Here's how the part is built. I have some questions about the finished solid (model axes, mm). A direction names the side the tool comes from. Round coordinates to 2 decimals unless told otherwise and drop trailing zeros. Write each loop counter-clockwise with the first axis right and the second up, starting at its lowest first coordinate (ties: lowest second). Pieces come first, ordered by that corner, then holes. Notation, with made-up numbers: M -27,-20 L 2,-20 A6 ccw 2,-15 Z; hole C -28.75,81 d7. An arc over 180 degrees is marked long. Use a Markdown table: item, result. Add a question column.
```python
from build123d import *

# Parameters (mm, degrees)
F0_W     = 12
F0_H     = 12
F1_DEPTH = 2
F2_R     = 1.5
F3_DEPTH = 10
F4_W     = 10
F4_H     = 10
F5_DEPTH = 1


with BuildPart() as f1:
    # F0 (on Top) → F1 (new body)
    with BuildSketch(Plane.XY):
        Rectangle(F0_W, F0_H)
    extrude(amount=F1_DEPTH)

    # F2 (on face) → F3 (join)
    with BuildSketch(Plane.XY.offset(2)):
        Circle(F2_R)
    extrude(amount=F3_DEPTH)

    # F4 (on face) → F5 (cut)
    with BuildSketch(Plane(origin=(0, 0, 0), x_dir=(1, 0, 0), z_dir=(0, 0, -1))):
        Rectangle(F4_W, F4_H)
    extrude(amount=-F5_DEPTH, mode=Mode.SUBTRACT)


solid = f1.part
```
Item 1: If we mould it in two halves opening along Y, with no side actions, what happens to faces 1 (the face through (-0.1, 5, 0.5)), 2 (the face through (-1.5, 0.07, 6.93)), 3 (the face through (-6, 0, 1))? For each: +Y half, -Y half, draft (parallel to the pull), parting line (faces both ways), or undercut.
Item 2: Imagine slicing it at A-A on y = 0. List the corners of the cut face in (x, z) for me.
Item 3: I need wall thicknesses on probe 1 along Z at (x, y) = (4, 4.75); probe 2 along Z at (x, y) = (-1, 5.25); probe 3 along X at (y, z) = (-0.25, 11.25). Which ranges of each line are inside material? Lowest first, please. Write a range as from..to.
Item 4: For pin 1 Ø1.5 at (x, z) = (-0.5, 3) entering from +Y; pin 2 Ø4 at (y, z) = (4.5, 9.5) entering from +X; pin 3 Ø1 at (x, z) = (1.5, 9.5) entering from -Y; pin 4 Ø5 at (x, y) = (-1, -1) entering from -Z, each with a flat end and sliding along its axis, tell me the tip position at first contact or that it passes through.
Item 5: Imagine slicing it at D-D on y = 3.5. List the corners of the cut face in (x, z) for me, plus the area to 3 significant figures.
Item 6: On a 3-axis mill with a long thin cutter (end or side, diameter ignored), from which of +Z, -Z, +X, -X, +Y, -Y can I reach the whole of each face in a straight line? I mean faces 4 (the face through (0, -6, 1)), 5 (the face through (0, 0, 1)), 6 (the face through (1.2, 1.4, 2)). Say none if no direction works.
Item 7: Imagine slicing it at C-C on z = 3.5. List the corners of the cut face in (x, y) for me.
The answers:
| question | item | result |
|---|---|---|
| 1 | face 1 | undercut |
| 1 | face 2 | parting line |
| 1 | face 3 | draft |
| 2 | outline | M -6,0 L -5,0 L -5,1 L 5,1 L 5,0 L 6,0 L 6,2 L 1.5,2 L 1.5,12 L -1.5,12 L -1.5,2 L -6,2 Z |
| 3 | probe 1 | 1..2 |
| 3 | probe 2 | 0..2 |
| 3 | probe 3 | -1.48..1.48 |
| 4 | pin 1 | y = 1.5 |
| 4 | pin 2 | through |
| 4 | pin 3 | y = -1.12 |
| 4 | pin 4 | z = 1 |
| 5 | outline | M -6,0 L -5,0 L -5,1 L 5,1 L 5,0 L 6,0 L 6,2 L -6,2 Z |
| 5 | area | 14.0 mm² |
| 6 | face 4 | +Z, -Z, +X, -X, -Y |
| 6 | face 5 | -Z |
| 6 | face 6 | +Z |
| 7 | outline | C 0,0 d3 |
